Part model, mm, in its own coordinate system. Face numbers are marked on the shaded views. Give positions to 0.01 mm unless a question says otherwise; leave off trailing zeros. Order: outer loops, then holes, each group sorted by start corner. A loop starts at its lowest first (then second) coordinate and runs counter-clockwise, first axis right, second up. Notation, with made-up numbers: (-7, -26.5) -> (26, -26.5) arc R17 ccw to (26, 1.5) -> close; hole circle Ø8 at (74, -20). An arc over 180 degrees is marked (long way). Write item = value, one per line. Start each with the question number.
Item 1: Band-saw the part on B-B on z = -48. Write the cut outline in (x, y).
Item 2: Band-saw the part on C-C on y = 4.1. Write the cut outline in (x, z).
Item 3: Drill centre lines: line 1 along X through (y, z) = (2.3, -10.02); line 2 along Z through (x, y) = (-5, 0.65); line 3 along X through (y, z) = (2.35, 7.5). Where is each one in solid material? Low to high.
Item 4: Flat gauge pins, fed straight in: P1, Ø3.5, axis at x = -5, z = -48, coming from the +Y side; P2, Ø5, axis at x = -16, z = -8, coming from the -Y side; P3, Ø1.6, axis at x = -48.5, z = -3.512, coming from the -Y side; P4, Ø1.5, axis at x = -50.5, y = 4, coming from the -Z side. Where does each tip first touch, or does it go through?
Item 5: Pull direction X, two halves, no side cores. Call the marked faces 1, 2, 3 and 4: +X half, -X half, draft (parallel to the pull), parting line (faces both ways), or undercut.
Item 6: Band-saw the part on D-D on x = -48.5. Write the cut outline in (y, z), plus the area to 3 significant figures.
Item 7: Band-saw the part on A-A on x = -5. Write the cut outline in (y, z).
Autodesk Inventor part; units mm, degrees
ref_plane "YZ Plane" through (0, 0, 0) normal (1, 0, 0) x (0, 1, 0)
ref_plane "XZ Plane" through (0, 0, 0) normal (0, 1, 0) x (-1, 0, 0)
ref_plane "XY Plane" through (0, 0, 0) normal (0, 0, 1) x (1, 0, 0)
sketch "Sketch3" plane through (0, 0, 0) normal (0, 1, 0) x (-1, 0, 0)
  line L0 (0, 0) -> (0, -60)
  line L1 (0, 0) -> (60, 0) construction
  line L2 (0, -60) -> (12.519, -60)
  line L3 (0, 0) -> (41, 0)
  line L4 (41, 0) -> (41, 7.5)
  arc A0 (56, 7.5) -> (41, 7.5) centre (48.5, 7.5) ccw
  line L5 (56, 7.5) -> (56, -16.519)
  line L6 (56, -16.519) -> (12.519, -60)
  line L7 (0, -30) -> (5, -30)
  line L8 (5, -60) -> (5, -48)
  line L9 (5, 0) -> (5, -12)
  circle A1 centre (5, -12) radius 1.5
  circle A2 centre (5, -48) radius 1.5
  circle A3 centre (48.5, 7.5) radius 4
  line L10 (48.5, 7.5) -> (48.5, -3.512)
  line L11 (48.5, -3.512) -> (48.5, -10.02)
  circle A4 centre (48.5, -3.512) radius 1
  circle A5 centre (48.5, -10.02) radius 1
  dimension "d6" = 60
  dimension "d7" = 90
  dimension "d8" = 12.519
  dimension "d9" = 41
  dimension "d10" = 7.5
  dimension "d11" = 15
  dimension "d13" = 24.019
  dimension "d18" = 5
  dimension "d19" = 12
  dimension "d20" = 12
  dimension "d21" = 3
  dimension "d22" = 3
  dimension "d25" = 8
  dimension "d26" = 11.012
  dimension "d27" = 6.508
  dimension "d28" = 2
  dimension "d29" = 2
extrude "Extrusion1" add sketch "Sketch3" along normal blind 3
sketch "Sketch6" plane through (0, 3, 0) normal (0, 1, 0) x (1, 0, 0)
  circle A0 centre (-48.5, -7.5) radius 4
  circle A1 centre (-5, 48) radius 1.5
  circle A2 centre (-5, 12) radius 1.5
  circle A3 centre (-48.5, 10.02) radius 1
  circle A4 centre (-48.5, 3.512) radius 1
  line L0 (0, 0) -> (0, 60)
  line L1 (0, 60) -> (-12.519, 60)
  line L2 (-12.519, 60) -> (-56, 16.519)
  line L3 (-56, 16.519) -> (-56, -7.5)
  arc A5 (-56, -7.5) -> (-41, -7.5) centre (-48.5, -7.5) ccw
  line L4 (-41, -7.5) -> (-41, 0)
  line L5 (-41, 0) -> (0, 0)
  line L6 (-56, 16.519) -> (-41, 16.519)
  line L7 (-41, -7.5) -> (-41, 0)
  line L8 (-41, 16.519) -> (-41, 0)
  circle A6 centre (-48.5, -7.5) radius 5.5
  line L9 (-48.5, 10.02) -> (-48.5, 11.52)
  circle A7 centre (-48.5, 11.52) radius 3
  line L10 (-54, -7.5) -> (-54, -4.5)
  line L11 (-43, -7.5) -> (-43, -4.5)
  line L12 (-43, -4.5) -> (-45.5349, 11.9762)
  line L13 (-54, -4.5) -> (-51.4651, 11.9762)
  dimension "d31" = 11
  dimension "d32" = 1.5
  dimension "d33" = 6
  dimension "d34" = 3
extrude "Extrusion3" add sketch "Sketch6" along normal blind 3 contours L4 A5 L3 L6 L8
properties part number "sideplateshaft_std"
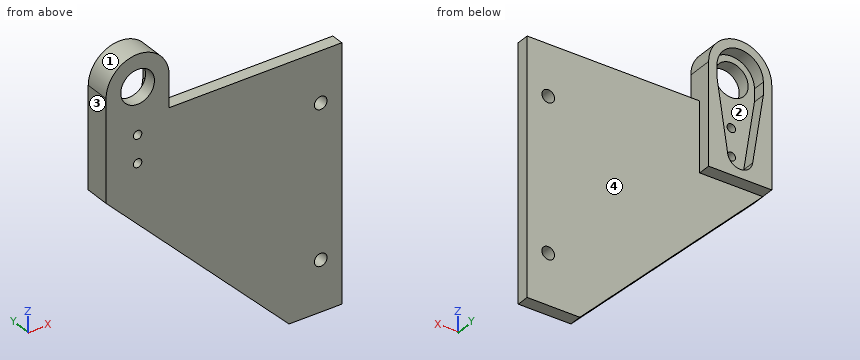
Values found:
q1.outline = (-24.52, 0) -> (-6.5, 0) -> (-6.5, 3) -> (-24.52, 3) -> close; (-3.5, 0) -> (0, 0) -> (0, 3) -> (-3.5, 3) -> close
q2.outline = (-56, -16.52) -> (-41, -16.52) -> (-41, 7.5) arc R7.5 ccw to (-56, 7.5) -> close; hole (-54, 4.5) -> (-51.47, -11.98) arc R3 ccw to (-45.53, -11.98) -> (-43, 4.5) -> (-43, 7.5) arc R5.5 ccw to (-54, 7.5) -> close
q3.line_1 = -56 to -49.5, -47.5 to 0
q3.line_2 = -60 to -49.5, -46.5 to -13.5, -10.5 to 0
q3.line_3 = -56 to -52.5, -44.5 to -41
q4.P1 = 3
q4.P2 = 0
q4.P3 = through
q4.P4 = -16.52
q5.face_1 = parting line
q5.face_2 = undercut
q5.face_3 = -X half
q5.face_4 = draft
q6.outline = (0, -24.02) -> (3, -24.02) -> (3, -16.52) -> (6, -16.52) -> (6, -14.52) -> (3, -14.52) -> (3, -11.02) -> (0, -11.02) -> close; (0, -9.02) -> (3, -9.02) -> (3, -4.51) -> (0, -4.51) -> close; (0, -2.51) -> (3, -2.51) -> (3, 3.5) -> (0, 3.5) -> close; (0, 11.5) -> (3, 11.5) -> (3, 13) -> (6, 13) -> (6, 15) -> (0, 15) -> close
q6.area = 93.1 mm^2
q7.outline = (0, -60) -> (3, -60) -> (3, -49.5) -> (0, -49.5) -> close; (0, -46.5) -> (3, -46.5) -> (3, -13.5) -> (0, -13.5) -> close; (0, -10.5) -> (3, -10.5) -> (3, 0) -> (0, 0) -> close
